Design review of the part shown in the three views and the two pictorial views. Dimensions are in mm from the part's minimum x, y and z. A direction names the side the tool comes from. Coordinates: 2 decimals unless noted, no trailing zeros. Order: outer loops, then holes, each group sorted by start corner. A loop starts at its lowest first (then second) coordinate and runs counter-clockwise, first axis right, second up. Notation, with made-up numbers: (-36.75, -22.5) -> (0.25, -22.5) arc R11 cw to (0.25, -9.5) -> close; hole circle Ø6 at (49.25, 6.5). An arc over 180 degrees is marked (long way). Answer as a JSON object with one key per item and string values. Group by question number.
1) Machinability: for the marked faces 4, 5 and 6, which of the approach directions +Z, -Z, +X, -X, +Y, -Y give a long, thin tool a straight path to every point of the face, cutting with its end or side? Answer none if there is none.
2) Add section B-B, the plane x = 12.5. Write out the cut boundary in (y, z), then the cut area to 3 significant figures.
3) Wall thickness on L1, parallel to Y at x = 12.5, z = 7.1; L2, parallel to Y at x = 15.25, z = 7 (1 decimal); L3, parallel to X at y = 9.25, z = 1.5 (1 decimal): over which ranges is each line inside the solid? List them lowest first.
4) For pin 1 (1.5 mm diameter, centred on y = 18, z = 5.5, fed in from -X); pin 2 (4 mm diameter, centred on x = 22.5, z = 2, fed in from +Y) (1 decimal); pin 3 (3 mm diameter, centred on x = 12, z = 0.5, fed in from +Y); pin 4 (1 mm diameter, centred on x = 12, y = 12, fed in from -Z), all flat-tipped, find the tip position at first contact; note any pin that passes through.
5) Draft analysis for pull direction Y (two halves, no side actions). For the marked faces 1, 2 and 3, state which applies: +Y half, -Y half, draft (parallel to the pull), parting line (faces both ways), or undercut.
6) Add section C-C, the plane z = 6. Write out the cut boundary in (x, y).
7) Add section A-A, the plane z = 1.5. Write out the cut boundary in (x, y).
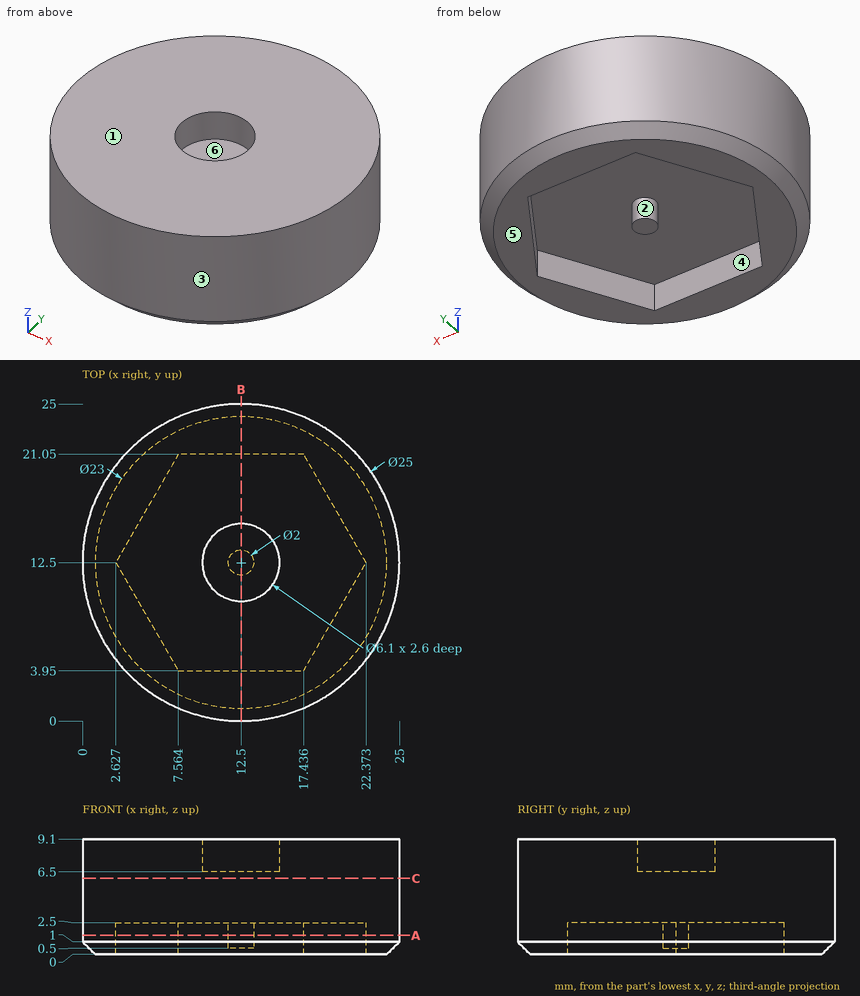
Output values:
{
 "1": {"face 4": "-Z", "face 5": "-Z, +X, -X, +Y, -Y", "face 6": "+Z"},
 "2": {"outline": "(0, 1) -> (1, 0) -> (3.95, 0) -> (3.95, 2.5) -> (11.5, 2.5) -> (11.5, 0.5) -> (13.5, 0.5) -> (13.5, 2.5) -> (21.05, 2.5) -> (21.05, 0) -> (24, 0) -> (25, 1) -> (25, 9.1) -> (15.55, 9.1) -> (15.55, 6.5) -> (9.45, 6.5) -> (9.45, 9.1) -> (0, 9.1) -> close", "area": "172 mm²"},
 "3": {"L1": "y = 0 to 9.45, 15.55 to 25", "L2": "y = 0.3 to 11.2, 13.8 to 24.7", "L3": "x = 0.4 to 4.5, 20.5 to 24.6"},
 "4": {"pin 1": "stops at x = 0.94", "pin 2": "stops at y = 22.1", "pin 3": "stops at y = 25", "pin 4": "stops at z = 0.5"},
 "5": {"face 1": "draft", "face 2": "undercut", "face 3": "parting line"},
 "6": {"outline": "circle Ø25 at (12.5, 12.5)"},
 "7": {"outline": "circle Ø25 at (12.5, 12.5); circle Ø2 at (12.5, 12.5); hole (2.63, 12.5) -> (7.56, 3.95) -> (17.44, 3.95) -> (22.37, 12.5) -> (17.44, 21.05) -> (7.56, 21.05) -> close"}
}
